Part model, mm, in its own coordinate system. Face numbers are marked on the shaded views. Coordinates: 2 decimals unless noted, no trailing zeros. Order: outer loops, then holes, each group sorted by start corner. A loop starts at its lowest first (then second) coordinate and runs counter-clockwise, first axis right, second up. Notation, with made-up numbers: (8, 44.25) - (42, 44.25) arc R20 ccw to (42, 57.25) - close; hole circle Ø11 at (29.5, 86.5). An arc over 180 degrees is marked (long way). Use a Markdown table: item, result. Add a question column.
1) Saw through at B-B on y = 8.75. List the corners of the cut face in (x, z), then the cut area to 3 significant figures.
2) Two-plate mould, pull along X, no slides. Class the marked faces 1 and 2: +X half, -X half, draft (parallel to the pull), parting line (faces both ways), or undercut.
3) Saw through at A-A on x = 0. List the corners of the cut face in (y, z).
4) Drop flat-ended pins along their axis: P1, Ø5, axis at x = 162.74, z = 0, coming from the -Y side; P2, Ø9.5, axis at y = 10.5, z = 5.5, coming from the -X side; P3, Ø8.5, axis at x = 0.5, y = 10.5, coming from the +Z side; P4, Ø10.5, axis at x = 0, z = 0, coming from the +Y side. Give the stop position or say it passes through.
5) Wall check: L1, parallel to X at y = 1.1, z = 0; L2, parallel to X at y = 12.75, z = -11; L3, parallel to X at y = 17.5, z = 6. Give the ranges that are in metal, low to high. Write a range as [from, to].
6) Saw through at D-D on x = -96. List the corners of the cut face in (y, z), then the cut area to 3 significant figures.
7) Saw through at C-C on z = 0. Count the separate pieces of the cut face and the enclosed holes in it, then the cut area to 3 significant figures.
```python
from build123d import *

# Parameters (mm, degrees)
CROQUIS1_R              = 4
SALIENTE_EXTRUIR1_DEPTH = 20
CROQUIS2_W              = 29.5
CROQUIS2_H              = 12
CORTAR_EXTRUIR1_DEPTH   = 180.732329924
CROQUIS3_W              = 41.22
CROQUIS3_H              = 42
CORTAR_EXTRUIR2_DEPTH   = 3
CHAFL_N1_SIZE           = 3
CROQUIS4_R              = 4
CORTAR_EXTRUIR3_DEPTH   = 176.518425627


with BuildPart() as part:
    # Croquis1 → Saliente-Extruir1 (new body)
    with BuildSketch(Plane(origin=(0, 0, 0), x_dir=(1, 0, 0), z_dir=(0, 1, 0))):
        with BuildLine():
            Line((20.61, 21), (22.109773483, 22.499773483))
            Line((22.109773483, 22.499773483), (25.109773482, 22.499825843))
            Line((25.109773482, 22.499825843), (161.820621985, 10.459829919))
            ThreePointArc((161.820621985, 10.459829919), (173.238204711, 0), (161.820621985, -10.459829919))
            Line((161.820621985, -10.459829919), (25.109773482, -22.499825843))
            Line((25.109773482, -22.499825843), (22.109773483, -22.499773483))
            Line((22.109773483, -22.499773483), (20.61, -21))
            Line((20.61, -21), (-20.61, -21))
            Line((-20.61, -21), (-22.109773483, -22.499773483))
            Line((-22.109773483, -22.499773483), (-25.109773482, -22.499825843))
            Line((-25.109773482, -22.499825843), (-161.820621985, -10.459829919))
            ThreePointArc((-161.820621985, -10.459829919), (-171.403039258, 0), (-161.820621985, 10.459829919))
            Line((-161.820621985, 10.459829919), (-25.109773482, 22.499825843))
            Line((-25.109773482, 22.499825843), (-22.109773483, 22.499773483))
            Line((-22.109773483, 22.499773483), (-20.61, 21))
            Line((-20.61, 21), (20.61, 21))
        make_face()
        with Locations(Location((-160.903039258, 0, 0), (0, 0, 270))):
            Circle(CROQUIS1_R, mode=Mode.SUBTRACT)
        with Locations(Location((162.738204711, 0, 0), (0, 0, 270))):
            Circle(CROQUIS1_R, mode=Mode.SUBTRACT)
    extrude(amount=SALIENTE_EXTRUIR1_DEPTH)

    # Croquis2 → Cortar-Extruir1 (cut, through all)
    with BuildSketch(Plane.XY.offset(21)):
        with Locations((-156.653039258, 10)):
            Rectangle(CROQUIS2_W, CROQUIS2_H)
        with Locations((158.488204711, 10)):
            Rectangle(CROQUIS2_W, CROQUIS2_H)
    extrude(amount=-CORTAR_EXTRUIR1_DEPTH, mode=Mode.SUBTRACT)

    # Croquis3 → Cortar-Extruir2 (cut)
    with BuildSketch(Plane(origin=(0, 20, 0), x_dir=(1, 0, 0), z_dir=(0, 1, 0))):
        Rectangle(CROQUIS3_W, CROQUIS3_H)
    extrude(amount=-CORTAR_EXTRUIR2_DEPTH, mode=Mode.SUBTRACT)

    # Chaflán1
    chafl_n1_edges = [part.edges().sort_by_distance(p)[0] for p in [
        (20.61, 20, 0),
        (-20.61, 20, 0),
    ]]
    chamfer(chafl_n1_edges, length=CHAFL_N1_SIZE - 0.0001)  # a hair under: the kernel refuses the full size

    # Croquis4 → Cortar-Extruir3 (cut, through all)
    with BuildSketch(Plane(origin=(0, 17, 0), x_dir=(1, 0, 0), z_dir=(0, 1, 0))):
        with Locations(Location((0, 0, 0), (0, 0, 270))):
            Circle(CROQUIS4_R)
    extrude(amount=-CORTAR_EXTRUIR3_DEPTH, mode=Mode.SUBTRACT)


solid = part.part
```
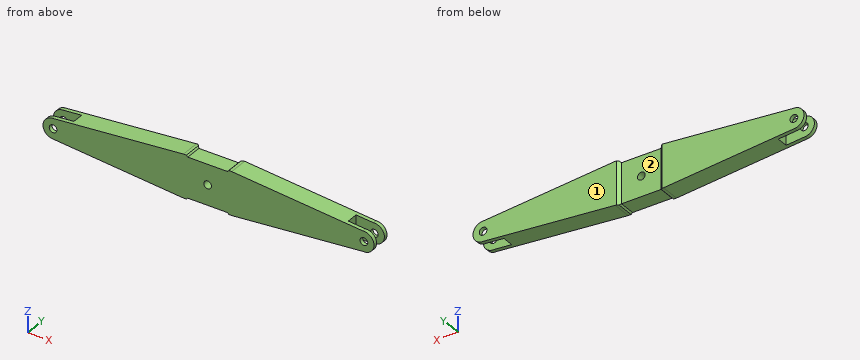
Results are:
| question | item | result |
|---|---|---|
| 1 | outline | (-141.9, -12.21) - (-25.11, -22.5) - (-22.11, -22.5) - (-20.61, -21) - (20.61, -21) - (22.11, -22.5) - (25.11, -22.5) - (143.74, -12.05) - (143.74, 12.05) - (25.11, 22.5) - (22.11, 22.5) - (20.61, 21) - (-20.61, 21) - (-22.11, 22.5) - (-25.11, 22.5) - (-141.9, 12.21) - close; hole circle Ø8 at (0, 0) |
| 1 | area | 10,200 mm2 |
| 2 | face 1 | draft |
| 2 | face 2 | undercut |
| 3 | outline | (0, -21) - (17, -21) - (17, -4) - (0, -4) - close; (0, 4) - (17, 4) - (17, 21) - (0, 21) - close |
| 4 | P1 | through |
| 4 | P2 | x = -141.9 |
| 4 | P3 | z = 21 |
| 4 | P4 | y = 17 |
| 5 | L1 | [-171.4, -164.9], [-156.9, -4], [4, 158.74], [166.74, 173.24] |
| 5 | L2 | [-141.9, 143.74] |
| 5 | L3 | [-169.52, -21.11], [21.11, 171.36] |
| 6 | outline | (0, -16.26) - (20, -16.26) - (20, 16.26) - (0, 16.26) - close |
| 6 | area | 650 mm2 |
| 7 | separate pieces | 6 |
| 7 | enclosed holes | 0 |
| 7 | area | 5,790 mm2 |
